Design review of the part shown in the three views and the two pictorial views. Dimensions are in mm from the part's minimum x, y and z. Coordinates: 2 decimals unless noted, no trailing zeros. Write each loop counter-clockwise with the first axis right and the second up, starting at its lowest first coordinate (ties: lowest second). Pieces come first, ordered by that corner, then holes. Notation, with made-up numbers: (80, 65.25) -> (85, 65.25) arc R32 cw to (85, 92.25) -> close; hole circle Ø7 at (57.25, 3.25). An arc over 180 degrees is marked (long way). Answer in a Markdown table with one row per item. Add a question column.
Item 1: Take a section at D-D, the plane z = 22.25. Write out the cut boundary in (x, y).
Item 2: To check wall thickness, follow line 1 (Y direction, x = 25.4, z = 4.5); line 2 (Z direction, x = 29.5, y = 29.5); line 3 (X direction, y = 9, z = 17.5). State the ranges of each line that lie inside material, in increasing order.
Item 3: Take a section at A-A, the plane y = 25.4. Write out the cut boundary in (x, z) (1 decimal), and give its area (3 significant figures).
Item 4: Take a section at C-C, the plane z = 15. Write out the cut boundary in (x, y) (1 decimal), and give its area (3 significant figures).
Item 5: Clearance check with flat-ended pins moving along their axes: P1, Ø12, axis at x = 28, z = 14.5, coming from the +Y side; P2, Ø1.5, axis at x = 6.5, z = 5, coming from the -Y side; P3, Ø3, axis at x = 16.5, z = 4, coming from the +Y side; P4, Ø2.5, axis at x = 25.4, y = 25.4, coming from the -Z side. State where each tip first meets the part, or that it passes through.
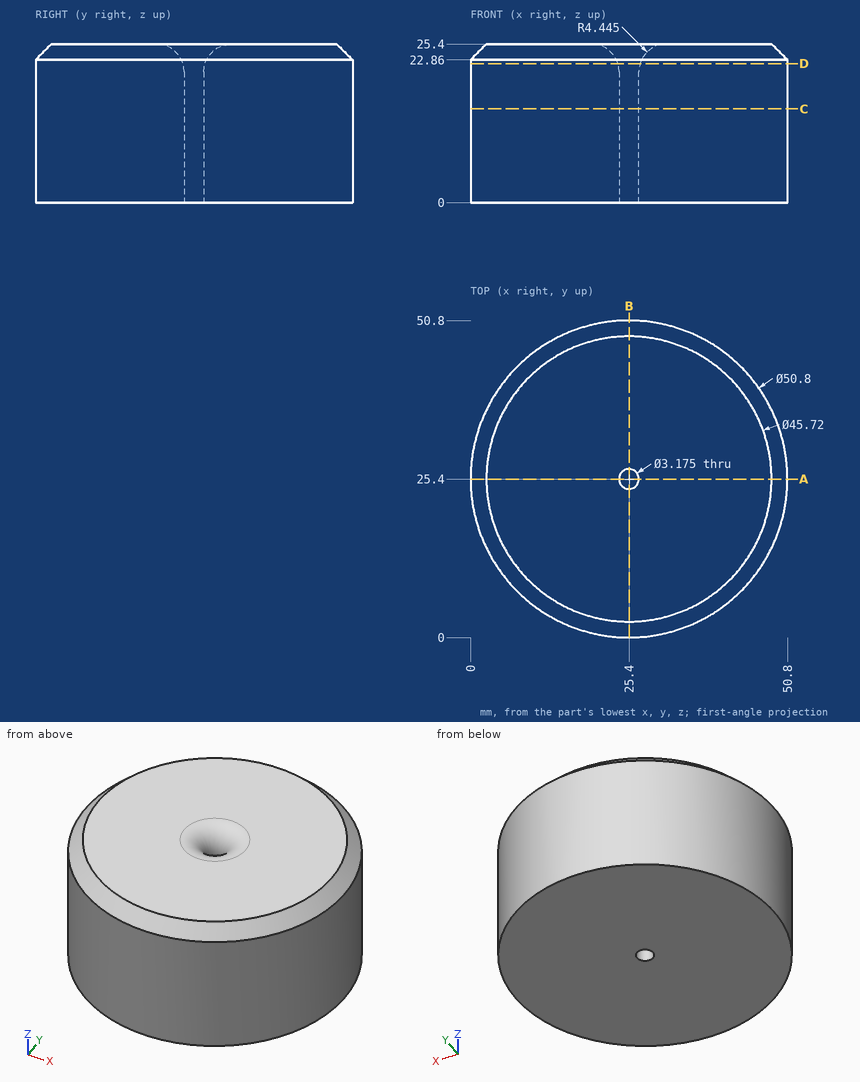
Answers:
| question | item | result |
|---|---|---|
| 1 | outline | circle Ø50.8 at (25.4, 25.4); hole circle Ø3.56 at (25.4, 25.4) |
| 2 | line 1 | y = 0 to 23.81, 26.99 to 50.8 |
| 2 | line 2 | z = 0 to 25.39 |
| 2 | line 3 | x = 6 to 44.8 |
| 3 | outline | (0, 0) -> (23.8, 0) -> (23.8, 21) arc R4.4 ccw to (19.4, 25.4) -> (2.5, 25.4) -> (0, 22.9) -> close; (27, 0) -> (50.8, 0) -> (50.8, 22.9) -> (48.3, 25.4) -> (31.4, 25.4) arc R4.4 ccw to (27, 21) -> close |
| 3 | area | 1,190 mm^2 |
| 4 | outline | circle Ø50.8 at (25.4, 25.4); hole circle Ø3.2 at (25.4, 25.4) |
| 4 | area | 2,020 mm^2 |
| 5 | P1 | stops at y = 50.8 |
| 5 | P2 | stops at y = 7.63 |
| 5 | P3 | stops at y = 49.7 |
| 5 | P4 | passes through |
